Design review of the part built by this model. Coordinates are the model's own, in mm. Round coordinates to 2 decimals unless told otherwise and drop trailing zeros. Write each loop counter-clockwise with the first axis right and the second up, starting at its lowest first coordinate (ties: lowest second). Pieces come first, ordered by that corner, then holes. Notation, with made-up numbers: M 25.5,66 L 72.5,66 A18 ccw 72.5,97 Z; hole C -29,-23.5 d8. An arc over 180 degrees is marked long. One line per question, with ' | ' between items. Start each with the question number.
Item 1: Insertion check: pin 1 Ø9.5 at (x, z) = (-15.51, 22.24) entering from -Y. The pin has a flat end and moves straight along its axis. Give the tip position at first contact, or say it passes through.
Item 2: Add section C-C, the plane x = 86. State the section outline as (y, z) points, and give its area (3 significant figures).
Item 3: Add section B-B, the plane y = 6.5. State the section outline as (x, z) points, and give its area (3 significant figures).
Item 4: For L1, parallel to Z at x = 35, y = 9; L2, parallel to Z at x = -10, y = 4.5, list the stretches that pass through material, from the lowest coordinate up.
Item 5: Add section A-A, the plane x = 39. State the section outline as (y, z) points, and give its area (3 significant figures).
```python
from build123d import *

# Parameters (mm, degrees)
SKETCH3_W           = 159.804878049
SKETCH3_H           = 120
BOSS_EXTRUDE1_DEPTH = 10
CUT_EXTRUDE1_DEPTH  = 20
SKETCH5_R           = 6
CUT_EXTRUDE3_DEPTH  = 20


with BuildPart() as part:
    # Sketch3 → Boss-Extrude1 (new body)
    with BuildSketch(Plane(origin=(0, 0, 0), x_dir=(1, 0, 0), z_dir=(0, 1, 0))):
        with Locations((34.390243903, -22.243902439)):
            Rectangle(SKETCH3_W, SKETCH3_H)
    extrude(amount=BOSS_EXTRUDE1_DEPTH)

    # Sketch4 → Cut-Extrude1 (cut)
    with BuildSketch(Plane(origin=(0, 10, 0), x_dir=(1, 0, 0), z_dir=(0, 1, 0))):
        Polygon((44.357270354, -22.243902439), (44.357270354, -32.248924449), (24.398521101, -32.248924449), (24.398521101, -12.268950417), (44.357270354, -12.268950417), align=None)
    extrude(amount=-CUT_EXTRUDE1_DEPTH, mode=Mode.SUBTRACT)

    # Sketch5 → Cut-Extrude3 (cut)
    with BuildSketch(Plane(origin=(0, 10, 0), x_dir=(1, 0, 0), z_dir=(0, 1, 0))):
        with Locations(Location((-15.512195122, -22.243902439, 0), (0, 0, 270))):
            Circle(SKETCH5_R)
        with Locations(Location((84.292682927, -22.243902439, 0), (0, 0, 270))):
            Circle(SKETCH5_R)
    extrude(amount=-CUT_EXTRUDE3_DEPTH, mode=Mode.SUBTRACT)


solid = part.part
```
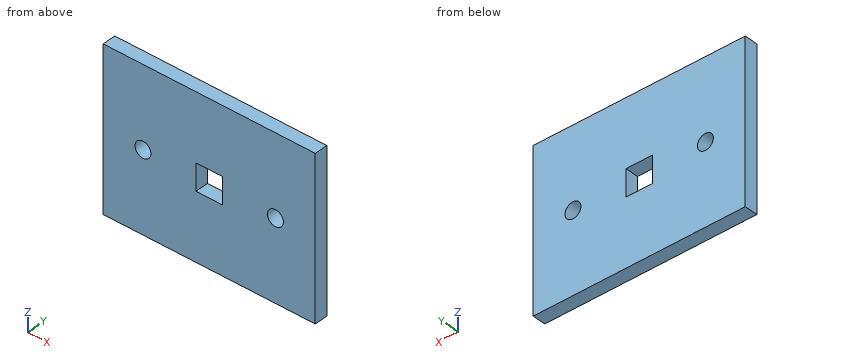
Computed values:
1) pin 1: passes through
2) outline: M 0,-37.76 L 10,-37.76 L 10,16.49 L 0,16.49 Z; M 0,28 L 10,28 L 10,82.24 L 0,82.24 Z | area: 1,080 mm^2
3) outline: M -45.51,-37.76 L 114.29,-37.76 L 114.29,82.24 L -45.51,82.24 Z; hole C -15.51,22.24 d12; hole M 24.4,12.27 L 44.36,12.27 L 44.36,32.25 L 24.4,32.25 Z; hole C 84.29,22.24 d12 | area: 18,600 mm^2
4) L1: z = -37.76 to 12.27, 32.25 to 82.24 | L2: z = -37.76 to 19.87, 24.61 to 82.24
5) outline: M 0,-37.76 L 10,-37.76 L 10,12.27 L 0,12.27 Z; M 0,32.25 L 10,32.25 L 10,82.24 L 0,82.24 Z | area: 1,000 mm^2
